Part model, mm, in its own coordinate system. Face numbers are marked on the shaded views. A direction names the side the tool comes from. Round coordinates to 2 decimals unless told otherwise and drop trailing zeros. Order: outer loops, then holes, each group sorted by start corner. A loop starts at its lowest first (then second) coordinate and runs counter-clockwise, first axis right, second up. Notation, with made-up numbers: (60, 88.5) - (73, 88.5) arc R21 cw to (73, 93.5) - close; hole circle Ø5 at (5.25, 6). An arc over 180 degrees is marked (long way). Answer as a JSON object with one key per item and string values.
```python
from build123d import *

# Parameters (mm, degrees)
SKETCH_1_W               = 60
SKETCH_1_H               = 32.5
SKETCH_1_R               = 4
SKETCH_1_R_2             = 3.3
SKETCH_1_W_2             = 34
SKETCH_1_H_2             = 6.5
EXTRUDE_1_DEPTH          = 20
SKETCH_4_R               = 5.5
CUT_EXTRUDE_1_DEPTH      = 49.541219597
CUT_EXTRUDE_1_DEPTH_BACK = 5
FILLET_1_R               = 1
FILLET_2_R               = 1
FILLET_4_R               = 1
FILLET_5_R               = 1
FILLET_6_R               = 1
FILLET_7_R               = 1
FILLET_8_R               = 1
FILLET_9_R               = 1
FILLET_10_R              = 1
FILLET_11_R              = 1
FILLET_12_R              = 1
SKETCH_5_R               = 3.3
CUT_EXTRUDE_2_DEPTH      = 89


with BuildPart() as part:
    # 草图1 → 凸台-拉伸1 (new body)
    with BuildSketch(Plane.XY):
        Rectangle(SKETCH_1_W, SKETCH_1_H)
        with Locations((0, 5.75)):
            Circle(SKETCH_1_R, mode=Mode.SUBTRACT)
        with Locations((-23, 5.75)):
            Circle(SKETCH_1_R_2, mode=Mode.SUBTRACT)
        with Locations((-23, -9.25)):
            Circle(SKETCH_1_R_2, mode=Mode.SUBTRACT)
        with Locations((23, -9.25)):
            Circle(SKETCH_1_R_2, mode=Mode.SUBTRACT)
        with Locations((23, 5.75)):
            Circle(SKETCH_1_R_2, mode=Mode.SUBTRACT)
        with Locations((0, 19.5)):
            Rectangle(SKETCH_1_W_2, SKETCH_1_H_2)
    extrude(amount=EXTRUDE_1_DEPTH)

    # 草图4 → 切除-拉伸1 (cut, two sides)
    with BuildSketch(Plane(origin=(0, 16.25, 0), x_dir=(1, 0, 0), z_dir=(0, 1, 0))) as cut_extrude_1_sk:
        with Locations(Location((-23, -10, 0), (0, 0, 270))):
            Circle(SKETCH_4_R)
        with Locations(Location((23, -10, 0), (0, 0, 270))):
            Circle(SKETCH_4_R)
    extrude(amount=CUT_EXTRUDE_1_DEPTH, mode=Mode.SUBTRACT)
    extrude(cut_extrude_1_sk.sketch, amount=-CUT_EXTRUDE_1_DEPTH_BACK, mode=Mode.SUBTRACT)

    # 圆角1
    fillet_1_edges = [part.edges().sort_by_distance(p)[0] for p in [
        (-17, 22.75, 10),
    ]]
    fillet(fillet_1_edges, radius=FILLET_1_R)

    # 圆角2
    fillet_2_edges = [part.edges().sort_by_distance(p)[0] for p in [
        (17, 22.75, 10),
    ]]
    fillet(fillet_2_edges, radius=FILLET_2_R)

    # 圆角4
    fillet_4_edges = [part.edges().sort_by_distance(p)[0] for p in [
        (30, 16.25, 10),
    ]]
    fillet(fillet_4_edges, radius=FILLET_4_R)

    # 圆角5
    fillet_5_edges = [part.edges().sort_by_distance(p)[0] for p in [
        (-30, 16.25, 10),
    ]]
    fillet(fillet_5_edges, radius=FILLET_5_R)

    # 圆角6
    fillet_6_edges = [part.edges().sort_by_distance(p)[0] for p in [
        (-17, 19, 20),
        (0, 22.75, 20),
        (-16.707106781, 22.457106781, 20),
        (17, 19, 20),
        (16.707106781, 22.457106781, 20),
    ]]
    fillet(fillet_6_edges, radius=FILLET_6_R)

    # 圆角7
    fillet_7_edges = [part.edges().sort_by_distance(p)[0] for p in [
        (-17, 19, 0),
        (0, 22.75, 0),
        (-16.707106781, 22.457106781, 0),
        (17, 19, 0),
        (16.707106781, 22.457106781, 0),
    ]]
    fillet(fillet_7_edges, radius=FILLET_7_R)

    # 圆角8
    fillet_8_edges = [part.edges().sort_by_distance(p)[0] for p in [
        (-22.5, 16.25, 20),
        (-30, -0.5, 20),
        (-29.707106781, 15.957106781, 20),
    ]]
    fillet(fillet_8_edges, radius=FILLET_8_R)

    # 圆角9
    fillet_9_edges = [part.edges().sort_by_distance(p)[0] for p in [
        (22.5, 16.25, 20),
        (30, -0.5, 20),
        (29.707106781, 15.957106781, 20),
    ]]
    fillet(fillet_9_edges, radius=FILLET_9_R)

    # 圆角10
    fillet_10_edges = [part.edges().sort_by_distance(p)[0] for p in [
        (22.5, 16.25, 0),
        (30, -0.5, 0),
        (29.707106781, 15.957106781, 0),
    ]]
    fillet(fillet_10_edges, radius=FILLET_10_R)

    # 圆角11
    fillet_11_edges = [part.edges().sort_by_distance(p)[0] for p in [
        (-22.5, 16.25, 0),
        (-30, -0.5, 0),
        (-29.707106781, 15.957106781, 0),
    ]]
    fillet(fillet_11_edges, radius=FILLET_11_R)

    # 圆角12
    fillet_12_edges = [part.edges().sort_by_distance(p)[0] for p in [
        (-30, -16.25, 10),
        (0, -16.25, 20),
        (-29.707106781, -16.25, 19.707106781),
        (30, -16.25, 10),
        (29.707106781, -16.25, 19.707106781),
        (29.707106781, -16.25, 0.292893219),
        (0, -16.25, 0),
        (-29.707106781, -16.25, 0.292893219),
    ]]
    fillet(fillet_12_edges, radius=FILLET_12_R)

    # 草图5 → 切除-拉伸2 (cut)
    with BuildSketch(Plane(origin=(0, 11.25, 0), x_dir=(1, 0, 0), z_dir=(0, 1, 0))):
        with Locations(Location((-23, -10, 0), (0, 0, 270))):
            Circle(SKETCH_5_R)
        with Locations(Location((23, -10, 0), (0, 0, 270))):
            Circle(SKETCH_5_R)
    extrude(amount=-CUT_EXTRUDE_2_DEPTH, mode=Mode.SUBTRACT)


solid = part.part
```
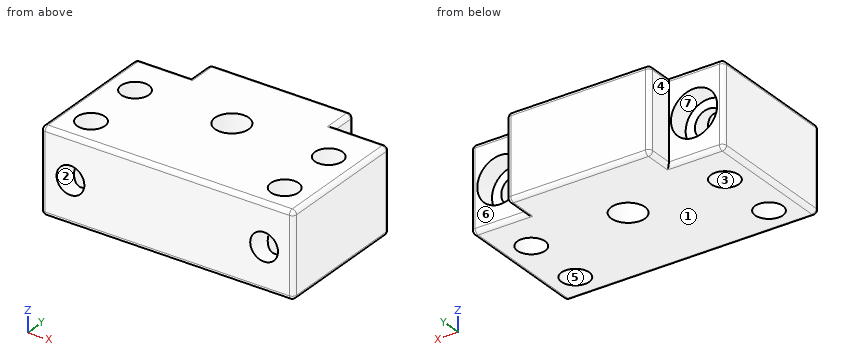
Item 1: Cut at A-A (x = 0). Write the cut outline in (y, z).
Taken from the geometry:
{"outline": "(-16.25, 1) arc R1 ccw to (-15.25, 0) - (1.75, 0) - (1.75, 20) - (-15.25, 20) arc R1 ccw to (-16.25, 19) - close; (9.75, 0) - (21.75, 0) arc R1 ccw to (22.75, 1) - (22.75, 19) arc R1 ccw to (21.75, 20) - (9.75, 20) - close"}
Item 2: Cut at C-C (x = 23). State how many separate pieces and enclosed holes the cut face has, plus the area to 3 significant figures.
Taken from the geometry:
{"separate pieces": "6", "enclosed holes": "0", "area": "236 mm2"}
Item 3: Cut at B-B (y = 12). Write the cut outline in (x, z).
Taken from the geometry:
{"outline": "(-30, 1) arc R1 ccw to (-29, 0) - (29, 0) arc R1 ccw to (30, 1) - (30, 19) arc R1 ccw to (29, 20) - (-29, 20) arc R1 ccw to (-30, 19) - close; hole circle Ø11 at (-23, 10); hole circle Ø11 at (23, 10)"}
Item 4: Probe L1, parallel to Y at x = -23, z = 17; L2, parallel to X at y = -9.25, z = 7.25; L3, parallel to Y at x = 23, z = 14.5. List the from-to ranges inside material, lowest first. Write a range as from..to.
Taken from the geometry:
{"L1": "-16.25..-12.55, -5.95..2.45, 9.05..16.25", "L2": "-30..-26.3, -19.7..19.7, 26.3..30", "L3": "-16.25..-12.55, -5.95..2.45, 9.05..11.25"}
Item 5: Drop flat-ended pins along their axis: P1, Ø10.5, axis at x = -23, z = 10, coming from the +Y side; P2, Ø6, axis at y = 18.5, z = 8, coming from the -X side; P3, Ø7, axis at x = 0, y = 5.75, coming from the -Z side; P4, Ø10, axis at x = -22.5, z = 3, coming from the +Y side. Give the stop position or say it passes through.
Taken from the geometry:
{"P1": "y = 11.25", "P2": "x = -29.97", "P3": "through", "P4": "y = 16.25"}
Item 6: Cut at D-D (z = 2.5). Write the cut outline in (x, y), plus the area to 3 significant figures.
Taken from the geometry:
{"outline": "(-30, -15.25) arc R1 ccw to (-29, -16.25) - (29, -16.25) arc R1 ccw to (30, -15.25) - (30, 15.25) arc R1 ccw to (29, 16.25) - (17, 16.25) - (17, 21.75) arc R1 ccw to (16, 22.75) - (-16, 22.75) arc R1 ccw to (-17, 21.75) - (-17, 16.25) - (-29, 16.25) arc R1 ccw to (-30, 15.25) - close; hole circle Ø6.6 at (-23, -9.25); hole circle Ø6.6 at (-23, 5.75); hole circle Ø8 at (0, 5.75); hole circle Ø6.6 at (23, -9.25); hole circle Ø6.6 at (23, 5.75)", "area": "1,980 mm2"}
Item 7: Tool access for the marked faces 4, 5, 6 and 7: list every direction of +Z, -Z, +X, -X, +Y, -Y with a clear straight run to the whole face (end or side of a thin tool).
Taken from the geometry:
{"face 4": "+Z, -Z, -X, +Y", "face 5": "+Z, -Z", "face 6": "+Z, -Z, +X, +Y", "face 7": "+Y"}
Item 8: Two-plate mould, pull along Z, no slides. Class the marked faces 1, 2 and 3: pulls with the +Z half, pulls with the -Z half, needs draft (parallel to the pull), parting line crosses it, or undercut.
Taken from the geometry:
{"face 1": "pulls with the -Z half", "face 2": "undercut", "face 3": "needs draft"}
